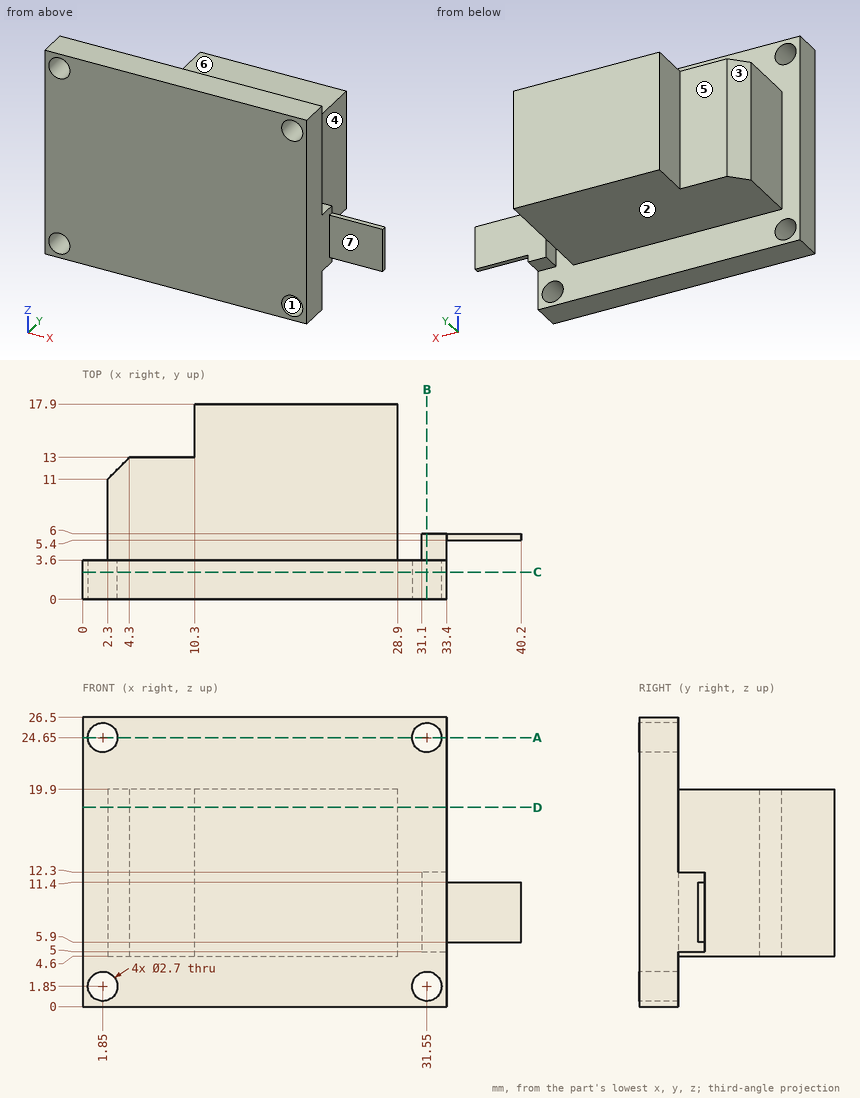
Here's the drawing with two shaded views (mm, measured from the low corner). I have some questions. A direction names the side the tool comes from. Give positions to 0.01 mm unless a question says otherwise; leave off trailing zeros. Write each loop counter-clockwise with the first axis right and the second up, starting at its lowest first coordinate (ties: lowest second). Pieces come first, ordered by that corner, then holes. Notation, with made-up numbers: (29, -11.75) -> (67, -11.75) arc R20 ccw to (67, 16.25) -> close; hole circle Ø1 at (-29, -28.75). An arc over 180 degrees is marked (long way). Answer as a JSON object with one key per item and string values. Group by question number.
Item 1: Please list where these lines run through material, in increasing order: line 1 (Z direction, x = 31.55, y = 1.45); line 2 (X direction, y = 1.4, z = 24.65); line 3 (Z direction, x = 28, y = 12). Write a range as [from, to].
Item 2: Suppose I cut it at A-A (z = 24.65). Please give me the cut outline in (x, y).
Item 3: Suppose I cut it at C-C (y = 2.5). Please give me the cut outline in (x, z).
Item 4: We'd pull the mould along Z, two halves only. Please class the marked faces 1, 2 and 3: +Z half, -Z half, draft (parallel to the pull), parting line (faces both ways), or undercut.
Item 5: Suppose I cut it at D-D (z = 18.25). Please give me the cut outline in (x, y), plus the area to 3 significant figures.
Item 6: For the marked faces 4, 5, 6 and 7, which set-ups out of +Z, -Z, +X, -X, +Y, -Y let a thin tool reach every point of the face, with its end or its side?
Item 7: Suppose I cut it at B-B (x = 31.55). Please give me the cut outline in (y, z), plus the area to 3 significant figures.
Item 8: I'm going to push flat-ended pins straight in: P1, Ø5, axis at x = 5.5, z = 17, coming from the -Y side; P2, Ø5, axis at y = 1.5, z = 15, coming from the +X side; P3, Ø4, axis at y = 11.5, z = 21.5, coming from the -X side; P4, Ø3, axis at x = 31.55, z = 24.65, coming from the +Y side. Where does each tip first touch, or does it pass through?
Findings:
{
 "1": {"line 1": "z = [0, 0.5], [3.2, 23.3], [26, 26.5]", "line 2": "x = [0, 0.5], [3.2, 30.2], [32.9, 33.4]", "line 3": "z = [4.6, 19.9]"},
 "2": {"outline": "(0, 0) -> (0.5, 0) -> (0.5, 3.6) -> (0, 3.6) -> close; (3.2, 0) -> (30.2, 0) -> (30.2, 3.6) -> (3.2, 3.6) -> close; (32.9, 0) -> (33.4, 0) -> (33.4, 3.6) -> (32.9, 3.6) -> close"},
 "3": {"outline": "(0, 0) -> (33.4, 0) -> (33.4, 26.5) -> (0, 26.5) -> close; hole circle Ø2.7 at (1.85, 1.85); hole circle Ø2.7 at (1.85, 24.65); hole circle Ø2.7 at (31.55, 1.85); hole circle Ø2.7 at (31.55, 24.65)"},
 "4": {"face 1": "undercut", "face 2": "-Z half", "face 3": "draft"},
 "5": {"outline": "(0, 0) -> (33.4, 0) -> (33.4, 3.6) -> (28.9, 3.6) -> (28.9, 17.9) -> (10.3, 17.9) -> (10.3, 13) -> (4.3, 13) -> (2.3, 11) -> (2.3, 3.6) -> (0, 3.6) -> close", "area": "459 mm²"},
 "6": {"face 4": "+Z, -Z, +Y", "face 5": "+Z, -Z, -X, +Y", "face 6": "+Z, +X, -X, +Y", "face 7": "+Z, -Z, +X, -Y"},
 "7": {"outline": "(0, 0) -> (3.6, 0) -> (3.6, 0.5) -> (0, 0.5) -> close; (0, 3.2) -> (3.6, 3.2) -> (3.6, 5) -> (6, 5) -> (6, 12.3) -> (3.6, 12.3) -> (3.6, 23.3) -> (0, 23.3) -> close; (0, 26) -> (3.6, 26) -> (3.6, 26.5) -> (0, 26.5) -> close", "area": "93.5 mm²"},
 "8": {"P1": "stops at y = 0", "P2": "stops at x = 33.4", "P3": "stops at x = 2.3", "P4": "stops at y = 3.6"}
}
